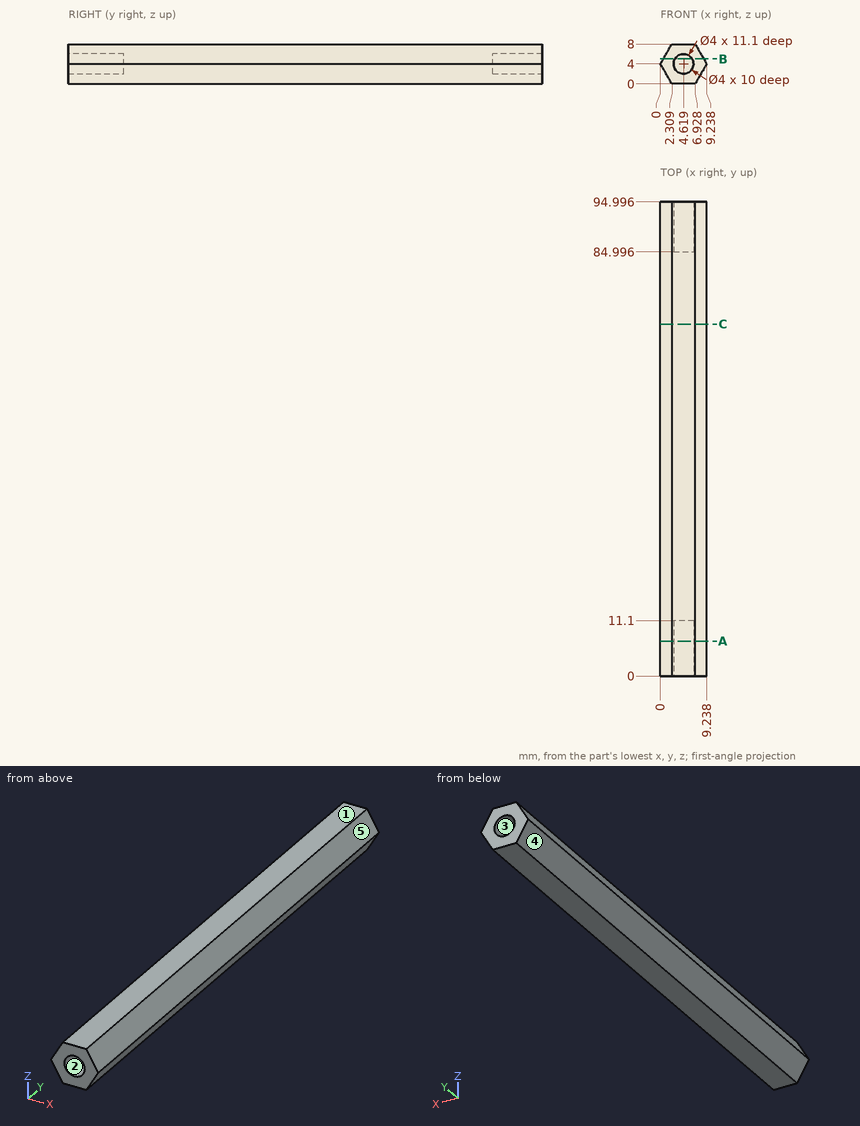
Source: three-view drawing plus pictorial views. Frame: mm from the lowest corner of the part. A direction names the side the tool comes from. Coordinates: 2 decimals unless noted, no trailing zeros. Write each loop counter-clockwise with the first axis right and the second up, starting at its lowest first coordinate (ties: lowest second). Pieces come first, ordered by that corner, then holes. Notation, with made-up numbers: (45.5, 85) -> (55.5, 85) arc R28 cw to (55.5, 118) -> close; hole circle Ø7 at (67.25, 72). An arc over 180 degrees is marked (long way). Write each question's results on one line, items separated by ' | '.
Item 1: Pin query (flat end, axial travel): pin 1 Ø1.5 at (x, y) = (1, 31.5) entering from -Z; pin 2 Ø2 at (x, z) = (5, 4.5) entering from -Y; pin 3 Ø2 at (x, z) = (4, 4.5) entering from +Y. Return the tip coordinate at first contact, or that it passes through.
Conclusion:
pin 1: stops at z = 0.97 | pin 2: stops at y = 11.1 | pin 3: stops at y = 85
Item 2: Section query C-C on y = 70.5. Return loops of the section in (x, z), plus the area to 3 significant figures.
Conclusion:
outline: (0, 4) -> (2.31, 0) -> (6.93, 0) -> (9.24, 4) -> (6.93, 8) -> (2.31, 8) -> close | area: 55.4 mm^2
Item 3: Mould query, pull axis X, two halves, no side actions, for the marked faces 3, 4 and 5. Classes: +X half, -X half, draft (parallel to the pull), parting line (faces both ways), or undercut.
Conclusion:
face 3: undercut | face 4: -X half | face 5: +X half
Item 4: Material intervals for probe 1 along X at (y, z) = (91, 4); probe 2 along X at (y, z) = (52.5, 1.25); probe 3 along X at (y, z) = (42.5, 5.75), sorted ascending.
Conclusion:
probe 1: x = 0 to 2.62, 6.62 to 9.24 | probe 2: x = 1.59 to 7.65 | probe 3: x = 1.01 to 8.23
Item 5: Section query A-A on y = 7. Return loops of the section in (x, z).
Conclusion:
outline: (0, 4) -> (2.31, 0) -> (6.93, 0) -> (9.24, 4) -> (6.93, 8) -> (2.31, 8) -> close; hole circle Ø4 at (4.62, 4)
Item 6: Section query B-B on z = 5. Return loops of the section in (x, y), plus the area to 3 significant figures.
Conclusion:
outline: (0.58, 0) -> (2.89, 0) -> (2.89, 11.1) -> (6.35, 11.1) -> (6.35, 0) -> (8.66, 0) -> (8.66, 95) -> (6.35, 95) -> (6.35, 85) -> (2.89, 85) -> (2.89, 95) -> (0.58, 95) -> close | area: 695 mm^2
Item 7: Set-up query: the marked faces 1 and 2. Return all of +Z, -Z, +X, -X, +Y, -Y with unobstructed straight access to the full face (end or side cutting, diameter ignored); none if empty.
Conclusion:
face 1: +Z, +X, -X, +Y, -Y | face 2: -Y
